Check sheet for the modelled part. Datum: model origin and axes. Units: mm. A direction names the side the tool comes from. Give positions to 0.01 mm unless a question says otherwise; leave off trailing zeros. Order: outer loops, then holes, each group sorted by start corner. A loop starts at its lowest first (then second) coordinate and runs counter-clockwise, first axis right, second up. Notation, with made-up numbers: (62, -11) - (84, -11) arc R19 cw to (84, 13) - close; hole circle Ø10 at (-2.75, 7.5). An arc over 180 degrees is marked (long way). Answer in a Markdown table with one row per item.
from build123d import *

# Parameters (mm, degrees)
SKETCH016_W     = 44
SKETCH016_H     = 23.4
PAD009_DEPTH    = 7
THICKNESS003_T  = 1
SKETCH017_W     = 23.4
SKETCH017_H     = 1
POCKET005_DEPTH = 1
SKETCH018_R     = 2.3
POCKET006_DEPTH = 1


with BuildPart() as part:
    # Sketch016 → Pad009 (new body)
    with BuildSketch(Plane.XY):
        Rectangle(SKETCH016_W, SKETCH016_H)
    extrude(amount=PAD009_DEPTH)

    # Thickness003
    thickness003_openings = [part.faces().sort_by_distance(p)[0] for p in [
        (0, 0, 7),
    ]]
    offset(amount=THICKNESS003_T, openings=thickness003_openings)

    # Sketch017 (on Face7 of Thickness003) → Pocket005 (cut)
    with BuildSketch(Plane.YZ.offset(23)):
        with Locations((0, 6.5)):
            Rectangle(SKETCH017_W, SKETCH017_H)
    extrude(amount=-POCKET005_DEPTH, mode=Mode.SUBTRACT)

    # Sketch018 (on Face15 of Pocket005) → Pocket006 (cut)
    with BuildSketch(Plane(origin=(-23, 0, 0), x_dir=(0, -1, 0), z_dir=(-1, 0, 0))):
        with Locations((0, 7)):
            Circle(SKETCH018_R)
    extrude(amount=-POCKET006_DEPTH, mode=Mode.SUBTRACT)


solid = part.part
(1) Gauge pin test, flat end, axial feed: P1, Ø5, axis at x = -7.5, y = -5, coming from the +Z side. Record the tip position at first contact, or that the pin passes through.
Geometry says:
| item | result |
|---|---|
| P1 | z = 0 |
(2) Cross-section at C-C, the plane x = 2. Record the cut outline in (y, z).
Geometry says:
| item | result |
|---|---|
| outline | (-12.7, 0) arc R1 ccw to (-11.7, -1) - (11.7, -1) arc R1 ccw to (12.7, 0) - (12.7, 7) - (11.7, 7) - (11.7, 0) - (-11.7, 0) - (-11.7, 7) - (-12.7, 7) - close |
(3) Cross-section at A-A, the plane y = 0. Record the cut outline in (x, z), then the cut area to 3 significant figures.
Geometry says:
| item | result |
|---|---|
| outline | (-23, 0) arc R1 ccw to (-22, -1) - (22, -1) arc R1 ccw to (23, 0) - (23, 6) - (22, 6) - (22, 0) - (-22, 0) - (-22, 4.7) - (-23, 4.7) - close |
| area | 56.3 mm² |
(4) Cross-section at B-B, the plane z = 3.25. Record the cut outline in (x, y), then the cut area to 3 significant figures.
Geometry says:
| item | result |
|---|---|
| outline | (-23, -11.7) arc R1 ccw to (-22, -12.7) - (22, -12.7) arc R1 ccw to (23, -11.7) - (23, 11.7) arc R1 ccw to (22, 12.7) - (-22, 12.7) arc R1 ccw to (-23, 11.7) - close; hole (-22, -11.7) - (22, -11.7) - (22, 11.7) - (-22, 11.7) - close |
| area | 138 mm² |
(5) Mould release check, pull along X, two halves, no side actions. Record for faces 4 (the flat face through (22, 0, 3)), 5 (the cylindrical face through (-22.715, 12.399, 3.549)), 6 (the cylindrical face through (22.699, -12.415, 3.549)), 7 (the flat face through (22.5, -0.2, 6)): pulls with the +X half, pulls with the -X half, needs draft (parallel to the pull), parting line crosses it, or undercut.
Geometry says:
| item | result |
|---|---|
| face 4 | undercut |
| face 5 | pulls with the -X half |
| face 6 | pulls with the +X half |
| face 7 | needs draft |
(6) Thickness scan on L1, parallel to X at y = -4, z = 5; L2, parallel to Y at x = -2.5, z = 5; L3, parallel to Z at x = 21, y = -2. Record the ranges inside material, lowest first.
Geometry says:
| item | result |
|---|---|
| L1 | -23 to -22, 22 to 23 |
| L2 | -12.7 to -11.7, 11.7 to 12.7 |
| L3 | -1 to 0 |
(7) Access from +Z, -Z, +X, -X, +Y, -Y to the whole of each face (thin tool, end or side, straight path). Record for faces 1 (the cylindrical face through (-22.715, 0.164, -0.699)), 2 (the flat face through (0, -11.7, 3)), 3 (the cylindrical face through (-22.51, 0.05, 4.7)).
Geometry says:
| item | result |
|---|---|
| face 1 | -Z, -X, +Y, -Y |
| face 2 | +Z |
| face 3 | +Z, -X |
